Geometry check sheet. Reference: the model listing, model coordinates, mm. A direction names the side the tool comes from. Coordinates: 2 decimals unless noted, no trailing zeros. Order: outer loops, then holes, each group sorted by start corner. A loop starts at its lowest first (then second) coordinate and runs counter-clockwise, first axis right, second up. Notation, with made-up numbers: (-38, -15.75) - (5, -15.75) arc R20 cw to (5, 3.25) - close; hole circle Ø6 at (87.25, 66). An arc over 180 degrees is marked (long way). Use CSV: the item, a comma, the result in double quotes. Start each with the question number.
1) Tool access check on faces 4 (the flat face through (6, 9, 2)), 5 (the cylindrical face through (5.014, 0.165, 21.246)). Record the directions out of +Z, -Z, +X, -X, +Y, -Y that give a thin tool (end or side, any length) a straight path to the whole face; none if there is none.
2) Depth check by flat-ended pin: P1, Ø12, axis at y = -12.37, z = 12.37, coming from the -X side; P2, Ø3, axis at y = -31, z = 0, coming from the -X side; P3, Ø4, axis at x = 3, z = 11, coming from the +Y side; P4, Ø2, axis at x = 9.5, z = -2.5, coming from the +Y side. Enter the tip coordinate at first touch or a pass-through.
3) Sectioned sample at B-B, the plane x = 14.5. Record the cut outline in (y, z).
4) Draft check along Z on faces 1 (the cylindrical face through (1.521, 15.875, 28.039)), 2 (the flat face through (0, -17, 20)), 3 (the cylindrical face through (20.09, -11.59, 0.51)). Enter one of: released by +Z, released by -Z, zero draft, split by the parting line, or undercut.
5) Sectioned sample at A-A, the plane z = 0. Count the separate pieces of the cut face and the enclosed holes in it, and give its area (3 significant figures).
6) Sectioned sample at D-D, the plane x = 7.75. Record the cut outline in (y, z).
7) Thickness scan on probe 1 along X at (y, z) = (10, 16.5); probe 2 along X at (y, z) = (2, 26.5); probe 3 along Y at (x, z) = (9, -7). Record the ranges inside material, lowest first. Write a range as [from, to].
from build123d import *

# Parameters (mm, degrees)
CHAMFER_1_SIZE           = 0.5
SKETCH_2_R               = 3.75
CUT_EXTRUDE_1_DEPTH      = 10
PATTERN_CIRCULAR_1_COUNT = 6
SKETCH_6_OUTSIDE_W       = 88.454
SKETCH_6_OUTSIDE_H       = 88.454
SKETCH_6_OUTSIDE_R       = 12.5
CUT_EXTRUDE_2_DEPTH      = 9.5
CHAMFER_2_SIZE           = 0.5


with BuildPart() as part:
    # 草图1 → 旋转1 (revolve)
    with BuildSketch(Plane.XY):
        Polygon((0, 33.5), (0, 25.5), (4, 25.5), (4, 9), (6, 9), (6, 10), (22, 10), (22, 13.5), (20.7, 13.5), (20.7, 11.6), (19.5, 11.6), (19.5, 13.5), (6, 13.5), (6, 27.5), (3, 27.5), (3, 33.5), align=None)
    revolve(axis=Axis((0, 0, 0), (1, 0, 0)))

    # 倒角1
    chamfer_1_edges = [part.edges().sort_by_distance(p)[0] for p in [
        (3, -33.5, 0),
        (6, -27.5, 0),
        (22, -13.5, 0),
        (22, -10, 0),
        (4, -9, 0),
        (0, -25.5, 0),
        (0, -33.5, 0),
    ]]
    chamfer(chamfer_1_edges, length=CHAMFER_1_SIZE)

    # 草图2 → 切除-拉伸1 (cut)
    with BuildSketch(Plane(origin=(6, 0, 0), x_dir=(0, 0, -1), z_dir=(1, 0, 0))):
        with Locations((0, -17.5)):
            Circle(SKETCH_2_R)
        with Locations((0, 17.5)):
            Circle(SKETCH_2_R)
        with Locations((12.374368671, 12.374368671)):
            Circle(SKETCH_2_R)
        with Locations((17.5, 0)):
            Circle(SKETCH_2_R)
        with Locations((12.374368671, -12.374368671)):
            Circle(SKETCH_2_R)
        with Locations((-12.374368671, -12.374368671)):
            Circle(SKETCH_2_R)
        with Locations((-17.5, 0)):
            Circle(SKETCH_2_R)
        with Locations((-12.374368671, 12.374368671)):
            Circle(SKETCH_2_R)
    extrude(amount=-CUT_EXTRUDE_1_DEPTH, mode=Mode.SUBTRACT)

    # 草图5 → M3 螺纹孔1 (revolve, cut)
    with BuildSketch(Plane(origin=(3, 31, 0), x_dir=(0, 0, -1), z_dir=(0, 1, 0))):
        Polygon((0, 0), (0, 8.251075774), (1.25, 7.5), (1.25, 0), align=None)
    hole_wizard_m3_1 = revolve(axis=Axis((9.35, 31, 0), (-1, 0, 0)), mode=Mode.SUBTRACT)

    # 阵列(圆周)1: M3 螺纹孔1 ×6 about axis
    pattern_circular_1_axis = Axis((0, 0, 0), (1, 0, 0))
    for i in range(1, PATTERN_CIRCULAR_1_COUNT):
        add(hole_wizard_m3_1.rotate(pattern_circular_1_axis, i * 360 / PATTERN_CIRCULAR_1_COUNT), mode=Mode.SUBTRACT)

    # 草图6 outside → 切除-拉伸2 (cut)
    with BuildSketch(Plane(origin=(22, 0, 0), x_dir=(0, 0, -1), z_dir=(1, 0, 0))):
        Rectangle(SKETCH_6_OUTSIDE_W, SKETCH_6_OUTSIDE_H)
        Circle(SKETCH_6_OUTSIDE_R, mode=Mode.SUBTRACT)
    extrude(amount=-CUT_EXTRUDE_2_DEPTH, mode=Mode.SUBTRACT)

    # 倒角2
    chamfer_2_edges = [part.edges().sort_by_distance(p)[0] for p in [
        (22, 0, 12.5),
    ]]
    chamfer(chamfer_2_edges, length=CHAMFER_2_SIZE)


solid = part.part
Evaluation:
1,face 4,"+X"
1,face 5,"+X, -X"
2,P1,"x = 4"
2,P2,"x = 0"
2,P3,"y = 32.25"
2,P4,"y = 13.42"
3,outline,"circle Ø25 at (0, 0); hole circle Ø20 at (0, 0)"
4,face 1,"undercut"
4,face 2,"zero draft"
4,face 3,"split by the parting line"
5,separate pieces,"6"
5,enclosed holes,"0"
5,area,"170 mm²"
6,outline,"circle Ø27 at (0, 0); hole circle Ø20 at (0, 0)"
7,probe 1,"[4, 6]"
7,probe 2,"[0, 6]"
7,probe 3,"[-11.54, -7.14], [7.14, 11.54]"
